Autodesk Inventor part; units mm, degrees
ref_plane "YZ Plane" through (0, 0, 0) normal (1, 0, 0) x (0, 1, 0)
ref_plane "XZ Plane" through (0, 0, 0) normal (0, 1, 0) x (-1, 0, 0)
ref_plane "XY Plane" through (0, 0, 0) normal (0, 0, 1) x (1, 0, 0)
sketch "Sketch1" plane through (0, 0, 0) normal (0, 1, 0) x (-1, 0, 0)
  line L0 (-4.6, 4.6) -> (4.6, 4.6)
  line L1 (4.6, 4.6) -> (4.6, -4.6)
  line L2 (4.6, -4.6) -> (-4.6, -4.6)
  line L3 (-4.6, -4.6) -> (-4.6, 4.6)
  point P0 (0, 0)
  dimension "d0" = 9.2
  dimension "d1" = 9.2
  dimension "d2" = 4.6
  dimension "d3" = 4.6
extrude "Extrusion1" add sketch "Sketch1" along normal blind 4.5
sketch "Sketch3" plane through (0, 0, 0) normal (0, -1, 0) x (1, 0, 0)
  line L0 (-4.6, -4.6) -> (4.6, -4.6)
  line L1 (-4.6, 4.6) -> (4.6, -4.6) construction
  line L2 (4.6, 4.6) -> (-4.6, -4.6) construction
  line L3 (1.3279, 2.3) -> (2.6558, 0)
  line L4 (2.6558, 0) -> (1.3279, -2.3)
  line L5 (1.3279, -2.3) -> (-1.3279, -2.3)
  line L6 (-1.3279, -2.3) -> (-2.6558, 0)
  line L7 (-2.6558, 0) -> (-1.3279, 2.3)
  line L8 (-1.3279, 2.3) -> (1.3279, 2.3)
  point P0 (0, 0)
  point P1 (0, 0)
  dimension "d7" = 4.6
extrude "Extrusion2" cut sketch "Sketch3" against normal blind 2.5
sketch "Sketch4" plane through (0, 4.5, 0) normal (0, 1, 0) x (1, 0, 0)
  circle A0 centre (0, 0) radius 1.3
  dimension "d10" = 2.6
extrude "Extrusion3" cut sketch "Sketch4" against normal blind 2
equation "\"d0\" = 2 * NutTrace"
equation "\"d1\" = d0"
equation "\"d4\" = ClassicThickness"
equation "\"d7\" = NutTrace"
equation "\"d8\" = NutThickness"
equation "\"d10\" = ServoScrewDiameterRequired"
equation "\"d11\" = MinimalThickness"
properties part number "ScrewHeadTrace"
Build history of the part. All positions in model axes, mm. A direction names the side the tool comes from. Coordinates: 2 decimals unless noted, no trailing zeros. Order: outer loops, then holes, each group sorted by start corner. A loop starts at its lowest first (then second) coordinate and runs counter-clockwise, first axis right, second up. Notation, with made-up numbers: (-14.75, 39) -> (-7.75, 39) arc R30 cw to (-7.75, 64) -> close; hole circle Ø11 at (69.25, -1). An arc over 180 degrees is marked (long way). Answer in a Markdown table with one row per item. Add a question column.
Q1. Mould opens along X. For faces 1 (the face through (-0.17, 3.51, -1.29)), 2 (the face through (4.6, 2, 0)), 3 (the face through (1.1, 4.5, 1.1)), 4 (the face through (1.98, 1.23, 1.17)) say: +X half, -X half, draft (parallel to the pull), parting line (faces both ways), or undercut.
Q2. Wall check: line 1 along Z through (x, y) = (0, 3.4); line 2 along Z through (x, y) = (1, 2.15). Give the ranges that are in metal, low to high. Write a range as [from, to].
Q3. Band-saw the part on B-B, the plane y = 0.6. List the corners of the cut face in (x, z), then the cut area to 3 significant figures.
Q4. Which spindle directions (+Z, -Z, +X, -X, +Y, -Y) get a long thin tool onto all of the face, cutting with end or side? Do faces 5 (the face through (1.1, 2.5, 1.1)), 6 (the face through (-4.6, 2, 0)). Say none if no direction does.
Q5. Band-saw the part on A-A, the plane x = 0. List the corners of the cut face in (y, z).
Q6. Band-saw the part on C-C, the plane z = -0.75. List the corners of the cut face in (x, y).
Q7. Drop a flat-ended pin along its axis: pin 1 (1.6 mm diameter, centred on x = 0, z = 0, fed in from -Y). Give the stop position or say it passes through.
Q8. Band-saw the part on D-D, the plane x = -2. List the corners of the cut face in (y, z), then the cut area to 3 significant figures.
Answers follow:
| question | item | result |
|---|---|---|
| 1 | face 1 | undercut |
| 1 | face 2 | +X half |
| 1 | face 3 | draft |
| 1 | face 4 | undercut |
| 2 | line 1 | [-4.6, -1.3], [1.3, 4.6] |
| 2 | line 2 | [-4.6, -2.3], [2.3, 4.6] |
| 3 | outline | (-4.6, -4.6) -> (4.6, -4.6) -> (4.6, 4.6) -> (-4.6, 4.6) -> close; hole (-2.66, 0) -> (-1.33, -2.3) -> (1.33, -2.3) -> (2.66, 0) -> (1.33, 2.3) -> (-1.33, 2.3) -> close |
| 3 | area | 66.3 mm^2 |
| 4 | face 5 | -Y |
| 4 | face 6 | +Z, -Z, -X, +Y, -Y |
| 5 | outline | (0, -4.6) -> (4.5, -4.6) -> (4.5, -1.3) -> (2.5, -1.3) -> (2.5, -2.3) -> (0, -2.3) -> close; (0, 2.3) -> (2.5, 2.3) -> (2.5, 1.3) -> (4.5, 1.3) -> (4.5, 4.6) -> (0, 4.6) -> close |
| 6 | outline | (-4.6, 0) -> (-2.22, 0) -> (-2.22, 2.5) -> (-1.06, 2.5) -> (-1.06, 4.5) -> (-4.6, 4.5) -> close; (1.06, 2.5) -> (2.22, 2.5) -> (2.22, 0) -> (4.6, 0) -> (4.6, 4.5) -> (1.06, 4.5) -> close |
| 7 | pin 1 | through |
| 8 | outline | (0, -4.6) -> (4.5, -4.6) -> (4.5, 4.6) -> (0, 4.6) -> (0, 1.14) -> (2.5, 1.14) -> (2.5, -1.14) -> (0, -1.14) -> close |
| 8 | area | 35.7 mm^2 |
